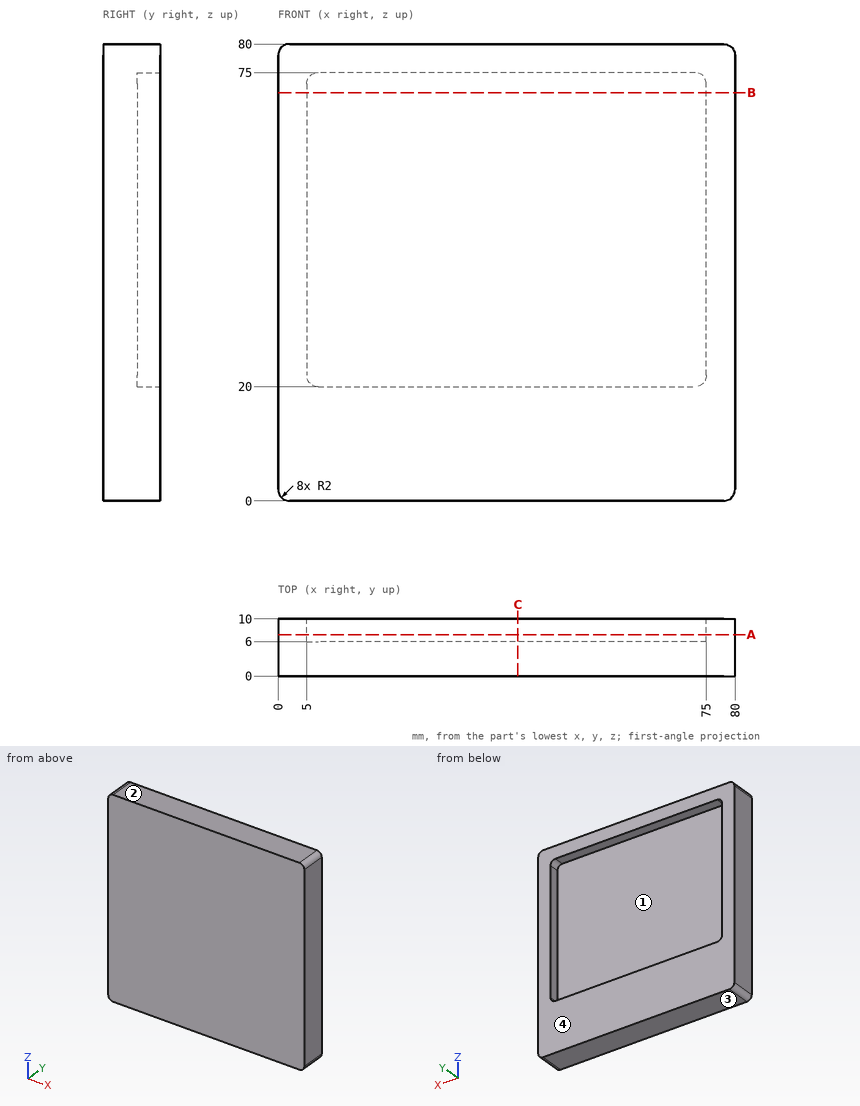
The drawing under review shows one solid part. Ordinate dimensions are in mm from its lowest x, y, z. Coordinates: 2 decimals unless noted, no trailing zeros. Loops run counter-clockwise (first coordinate to the right, second up) from the corner with the lowest first, then second, coordinate; pieces in that order, holes last.
Item 1: Draft analysis for pull direction Z (two halves, no side actions). For the marked faces 1, 2, 3 and 4, state which applies: pulls with the +Z half, pulls with the -Z half, needs draft (parallel to the pull), parting line crosses it, or undercut.
Completed:
face 1: undercut
face 2: pulls with the +Z half
face 3: pulls with the -Z half
face 4: needs draft
Item 2: Add section A-A (y = 7.25). Write out the cut boundary in (x, z).
Completed:
outline: (0, 2) arc R2 ccw to (2, 0) - (78, 0) arc R2 ccw to (80, 2) - (80, 78) arc R2 ccw to (78, 80) - (2, 80) arc R2 ccw to (0, 78) - close; hole (5, 22) arc R2 ccw to (7, 20) - (73, 20) arc R2 ccw to (75, 22) - (75, 73) arc R2 ccw to (73, 75) - (7, 75) arc R2 ccw to (5, 73) - close
Item 3: Add section B-B (z = 71.5). Write out the cut boundary in (x, y), and give its area (3 significant figures).
Completed:
outline: (0, 0) - (80, 0) - (80, 10) - (75, 10) - (75, 6) - (5, 6) - (5, 10) - (0, 10) - close
area: 520 mm2
Item 4: Wall thickness on L1, parallel to X at y = 9.25, z = 42; L2, parallel to Z at x = 41, y = 8.5; L3, parallel to Y at x = 39.5, z = 63: over which ranges is each line inside the solid? List them lowest first.
Completed:
L1: x = 0 to 5, 75 to 80
L2: z = 0 to 20, 75 to 80
L3: y = 0 to 6
Item 5: Clearance check with flat-ended pins moving along their axes: pin 1 (6 mm diameter, centred on y = 3.5, z = 30, fed in from -X); pin 2 (4 mm diameter, centred on x = 55, z = 48.5, fed in from +Y). State where each tip first meets the part, or that it passes through.
Completed:
pin 1: stops at x = 0
pin 2: stops at y = 6
Item 6: Add section C-C (x = 42). Write out the cut boundary in (y, z), and give its area (3 significant figures).
Completed:
outline: (0, 0) - (10, 0) - (10, 20) - (6, 20) - (6, 75) - (10, 75) - (10, 80) - (0, 80) - close
area: 580 mm2
